Input: part model. Units: mm. Frame: model coordinates. Coordinates: 2 decimals unless noted, no trailing zeros. Write each loop counter-clockwise with the first axis right and the second up, starting at its lowest first coordinate (ties: lowest second). Pieces come first, ordered by that corner, then holes. Notation, with made-up numbers: M 10,88.5 L 60,88.5 A38 ccw 60,127.5 Z; hole C 55.5,-33.75 d11. An arc over 180 degrees is marked long. Answer as a JSON object with one key per item and string values. Group by question number.
from build123d import *

# Parameters (mm, degrees)
SKETCH_1_W          = 58
SKETCH_1_H          = 36
EXTRUDE_1_DEPTH     = 3
SKETCH_2_W          = 52.5
SKETCH_2_H          = 30.5
CUT_EXTRUDE_1_DEPTH = 2
SKETCH_3_W          = 50
SKETCH_3_H          = 28
CUT_EXTRUDE_2_DEPTH = 2
FILLET_1_R          = 2
SKETCH_4_W          = 58
SKETCH_4_H          = 36
CUT_EXTRUDE_3_DEPTH = 1
FILLET_2_R          = 0.2
SKETCH_5_R          = 0.8
CUT_EXTRUDE_4_DEPTH = 1
SKETCH_6_R          = 0.6
CUT_EXTRUDE_5_DEPTH = 20.5


with BuildPart() as part:
    # 草图1 → 凸台-拉伸1 (new body)
    with BuildSketch(Plane.XY):
        Rectangle(SKETCH_1_W, SKETCH_1_H)
    extrude(amount=EXTRUDE_1_DEPTH)

    # 草图2 → 切除-拉伸1 (cut)
    with BuildSketch(Plane(origin=(0, 0, 0), x_dir=(-1, 0, 0), z_dir=(0, 0, -1))):
        Rectangle(SKETCH_2_W, SKETCH_2_H)
    extrude(amount=-CUT_EXTRUDE_1_DEPTH, mode=Mode.SUBTRACT)

    # 草图3 → 切除-拉伸2 (cut)
    with BuildSketch(Plane.XY.offset(3)):
        Rectangle(SKETCH_3_W, SKETCH_3_H)
    extrude(amount=-CUT_EXTRUDE_2_DEPTH, mode=Mode.SUBTRACT)

    # 圆角1
    fillet_1_edges = [part.edges().sort_by_distance(p)[0] for p in [
        (25, 14, 2.5),
        (25, -14, 2.5),
        (-25, -14, 2.5),
        (-25, 14, 2.5),
        (29, -18, 1.5),
        (-29, -18, 1.5),
        (-29, 18, 1.5),
        (29, 18, 1.5),
    ]]
    fillet(fillet_1_edges, radius=FILLET_1_R)

    # 草图4 → 切除-拉伸3 (cut)
    with BuildSketch(Plane(origin=(0, 0, 0), x_dir=(-1, 0, 0), z_dir=(0, 0, -1))):
        Rectangle(SKETCH_4_W, SKETCH_4_H)
    extrude(amount=-CUT_EXTRUDE_3_DEPTH, mode=Mode.SUBTRACT)

    # 圆角2
    fillet_2_edges = [part.edges().sort_by_distance(p)[0] for p in [
        (-26.25, 15.25, 1.5),
        (-26.25, -15.25, 1.5),
        (26.25, -15.25, 1.5),
        (26.25, 15.25, 1.5),
    ]]
    fillet(fillet_2_edges, radius=FILLET_2_R)

    # 草图5 → 切除-拉伸4 (cut)
    with BuildSketch(Plane.XY.offset(3)):
        with Locations((-27.5, 16.5)):
            Circle(SKETCH_5_R)
        with Locations((27.5, 16.5)):
            Circle(SKETCH_5_R)
        with Locations((27.5, -16.5)):
            Circle(SKETCH_5_R)
        with Locations((-27.5, -16.5)):
            Circle(SKETCH_5_R)
    extrude(amount=-CUT_EXTRUDE_4_DEPTH, mode=Mode.SUBTRACT)

    # 草图6 → 切除-拉伸5 (cut)
    with BuildSketch(Plane.XY.offset(2)):
        with Locations((-27.5, 16.5)):
            Circle(SKETCH_6_R)
        with Locations((27.5, 16.5)):
            Circle(SKETCH_6_R)
        with Locations((27.5, -16.5)):
            Circle(SKETCH_6_R)
        with Locations((-27.5, -16.5)):
            Circle(SKETCH_6_R)
    extrude(amount=-CUT_EXTRUDE_5_DEPTH, mode=Mode.SUBTRACT)


solid = part.part
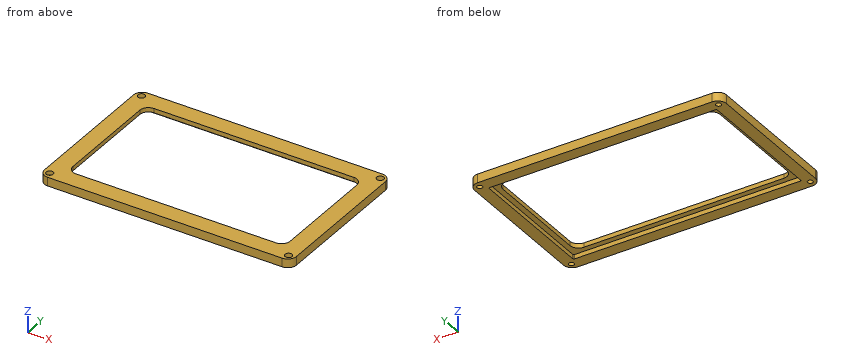
Q1. Section C-C, the plane y = -6. Return the cut outline in (x, z), and give its area (3 significant figures).
Q2. Section A-A, the plane x = -6. Return the cut outline in (y, z).
Q3. Line query: line 1 (Y direction, x = 23, z = 1.25); line 2 (X direction, y = 8, z = 2.5); line 3 (Y direction, x = 1.5, z = 2.3). Output: solid intervals per line, ascending. Write a range as from..to.
Q4. Section B-B, the plane z = 1.45. Return the cut outline in (x, y), and give its area (3 significant figures).
Filled in:
{
 "1": {"outline": "M -29,1 L -26.25,1 L -26.25,2 L -25,2 L -25,3 L -29,3 Z; M 25,2 L 26.25,2 L 26.25,1 L 29,1 L 29,3 L 25,3 Z", "area": "13.5 mm^2"},
 "2": {"outline": "M -18,1 L -15.25,1 L -15.25,2 L -14,2 L -14,3 L -18,3 Z; M 14,2 L 15.25,2 L 15.25,1 L 18,1 L 18,3 L 14,3 Z"},
 "3": {"line 1": "-18..-15.25, 15.25..18", "line 2": "-29..-25, 25..29", "line 3": "-18..-14, 14..18"},
 "4": {"outline": "M -29,-16 A2 ccw -27,-18 L 27,-18 A2 ccw 29,-16 L 29,16 A2 ccw 27,18 L -27,18 A2 ccw -29,16 Z; hole C -27.5,-16.5 d1.2; hole C -27.5,16.5 d1.2; hole M -26.25,-15.05 A0.2 ccw -26.05,-15.25 L 26.05,-15.25 A0.2 ccw 26.25,-15.05 L 26.25,15.05 A0.2 ccw 26.05,15.25 L -26.05,15.25 A0.2 ccw -26.25,15.05 Z; hole C 27.5,-16.5 d1.2; hole C 27.5,16.5 d1.2", "area": "479 mm^2"}
}
